Autodesk Inventor part; units mm, degrees
ref_plane "YZ Plane" through (0, 0, 0) normal (1, 0, 0) x (0, 1, 0)
ref_plane "XZ Plane" through (0, 0, 0) normal (0, 1, 0) x (-1, 0, 0)
ref_plane "XY Plane" through (0, 0, 0) normal (0, 0, 1) x (1, 0, 0)
sketch "Sketch1" plane through (0, 0, 0) normal (0, 0, 1) x (1, 0, 0)
  line L0 (15, 0) -> (25, 0)
  line L1 (25, 225) -> (0, 225)
  line L2 (0, 225) -> (0, 205)
  line L3 (25, 0) -> (25, 100)
  line L4 (25, 100) -> (50, 100)
  line L5 (50, 100) -> (50, 95)
  line L6 (50, 95) -> (55, 95)
  line L7 (55, 95) -> (55, 103)
  line L8 (53, 105) -> (30, 105)
  line L9 (25, 110) -> (25, 225)
  arc A0 (55, 103) -> (53, 105) centre (53, 103) ccw
  arc A1 (25, 110) -> (30, 105) centre (30, 110) ccw
  line L10 (0, 0) -> (0, 225)
  line L11 (15, 0) -> (15, 200)
  line L12 (10, 205) -> (0, 205)
  arc A2 (15, 200) -> (10, 205) centre (10, 200) ccw
  point P0 (20, 205)
  point P1 (55, 105)
  point P2 (25, 105)
  point P3 (15, 205)
  dimension "d1" = 10
  dimension "d2" = 225
  dimension "d3" = 20
  dimension "d4" = 20
  dimension "d6" = 100
  dimension "d7" = 25
  dimension "d8" = 5
  dimension "d9" = 5
  dimension "d10" = 10
  dimension "d11" = 2
  dimension "d12" = 5
  dimension "d28" = 205
  dimension "d29" = 5
revolve "Revolution1" add sketch "Sketch1" angle 360 about axis through (0, 0, 0) along (0, 1, 0)
sketch "Sketch2" plane through (0, 225, 0) normal (0, 1, 0) x (1, 0, 0)
  circle A0 centre (0, 0) radius 25
  line L0 (-12.5, 21.6506) -> (-12.5, -21.6506)
  line L1 (12.5, 0) -> (12.5, 21.6506)
  line L2 (12.5, 21.6506) -> (12.5, -21.6506)
  arc A1 (12.5, 21.6506) -> (-12.5, 21.6506) centre (0, 0) ccw
  arc A2 (-12.5, -21.6506) -> (12.5, -21.6506) centre (0, 0) ccw
  dimension "d14" = 12.5
extrude "Extrusion1" add sketch "Sketch2" along normal blind 30 contours L1 L2 A0 L0
sketch "Sketch3" plane through (12.5, 225, 21.6506) normal (1, 0, 0) x (0, 0, -1)
  line L0 (0, 0) -> (43.3013, 0)
  line L1 (43.3013, 0) -> (43.3013, 30)
  line L2 (0, 30) -> (-3.3494, 30)
  circle A0 centre (21.6506, 15) radius 5
  point P0 (21.6506, -225)
  dimension "d18" = 10
hole "Hole1" at (12.5, 240, 0) direction (-1, 0, 0) diameter 20 end through all
fillet "Fillet1" radius 2 2 edges at (-12.5, 225, 0) (12.5, 225, -10.8253)
fillet "Fillet2" radius 2 4 edges at (12.5, 255, -10.8253) (-12.5, 255, 0) (0, 255, 25) (0, 255, -25)
properties part number "Hydraulic fluid shield" material "Steel, High Strength, Low Alloy"
Input: part model. Units: mm. Frame: model coordinates. A direction names the side the tool comes from. Give positions to 0.01 mm unless a question says otherwise; leave off trailing zeros. Loops run counter-clockwise (first coordinate to the right, second up) from the corner with the lowest first, then second, coordinate; pieces in that order, holes last. Notation, with made-up numbers: (71, 89) -> (80, 89) arc R21 ccw to (80, 116) -> close; hole circle Ø8 at (74.5, 88). An arc over 180 degrees is marked (long way). Use a Markdown table: item, result.
Q1. First-contact query: P1, Ø22, axis at x = 2, z = 2.5, coming from the -Y side; P2, Ø11.5, axis at x = -21.5, z = 8, coming from the +Y side; P3, Ø3, axis at x = 29.5, z = 41.5, coming from the -Y side; P4, Ø8, axis at x = 12.5, z = -22.5, coming from the +Y side. Flat tips, straight axial feed; report the tip coordinate or a pass-through.
Entries:
| item | result |
|---|---|
| P1 | stops at y = 202.71 |
| P2 | stops at y = 225 |
| P3 | stops at y = 95 |
| P4 | stops at y = 255 |
Q2. Access query for faces 1 (the flat face through (0, 205, 0)), 2 (the flat face through (11, 0, 11)), 3 (the cylindrical face through (11.5, 166.6, 22.2)), 4 (the flat face through (-12.5, 231, -5)), 5 (the flat face through (19, 225, 0)). Directions: +Z, -Z, +X, -X, +Y, -Y. A direction counts if a zero-diameter tool reaches every point of the face in a straight line with its end or side. Return the directions, or none.
Entries:
| item | result |
|---|---|
| face 1 | -Y |
| face 2 | +Z, -Z, +X, -X, -Y |
| face 3 | +Y |
| face 4 | +Z, -Z, -X, +Y |
| face 5 | +Z, -Z, +X, +Y |
Q3. Section query A-A, the plane y = 240. Return the cut outline in (x, z).
Entries:
| item | result |
|---|---|
| outline | (-12.5, -21.65) arc R25 ccw to (12.5, -21.65) -> (12.5, -10) -> (-12.5, -10) -> close; (-12.5, 10) -> (12.5, 10) -> (12.5, 21.65) arc R25 ccw to (-12.5, 21.65) -> close |
Q4. Section query C-C, the plane y = 165.5. Return the cut outline in (x, z).
Entries:
| item | result |
|---|---|
| outline | circle Ø50 at (0, 0); hole circle Ø30 at (0, 0) |
Q5. Ray query, probe 1 along Z at (x, y) = (0, 96.35); probe 2 along Z at (x, y) = (0, 50); probe 3 along X at (y, z) = (102.5, 0). Return the intervals inside material, ascending. Write a range as from..to.
Entries:
| item | result |
|---|---|
| probe 1 | z = -55..-50, -25..-15, 15..25, 50..55 |
| probe 2 | z = -25..-15, 15..25 |
| probe 3 | x = -55..-15, 15..55 |
Q6. Pull-direction query (Y, two-part tool) for faces 6 (the flat face through (23, 105, 23)), 7 (the flat face through (-22.9, 100, 10.4)), 8 (the cylindrical face through (-0.18, 231.57, -5.38)); classes: pulls with the +Y half, pulls with the -Y half, needs draft (parallel to the pull), parting line crosses it, or undercut.
Entries:
| item | result |
|---|---|
| face 6 | pulls with the +Y half |
| face 7 | pulls with the -Y half |
| face 8 | undercut |
